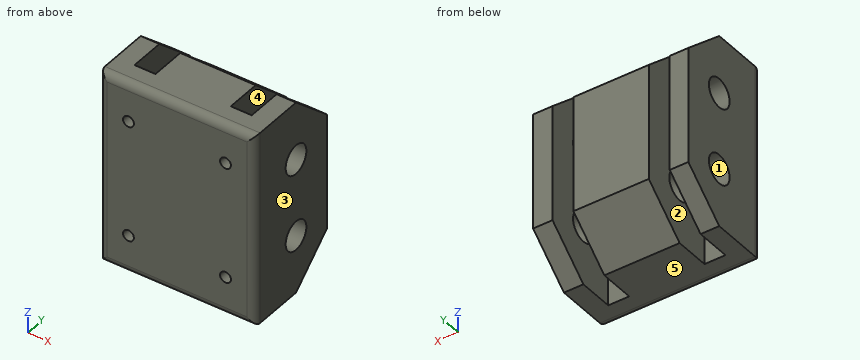
```python
from build123d import *

# Parameters (mm, degrees)
SKETCH1_W           = 63.5
SKETCH1_H           = 6.35
BOSS_EXTRUDE1_DEPTH = 50.8
BOSS_EXTRUDE2_DEPTH = 50.8
SKETCH10_W          = 6.858
SKETCH10_H          = 25.629031657
CUT_EXTRUDE1_DEPTH  = 88.854357354
LPATTERN3_COUNT     = 2
LPATTERN3_PITCH     = 31.496
SKETCH11_R          = 4.7625
CUT_EXTRUDE2_DEPTH  = 88.854357354
FILLET1_R           = 2.54
SKETCH19_R          = 1.778
CUT_EXTRUDE3_DEPTH  = 7.62


with BuildPart() as part:
    # Sketch1 → Boss-Extrude1 (new body)
    with BuildSketch(Plane(origin=(0, 0, 0), x_dir=(0, 0, -1), z_dir=(1, 0, 0))):
        with Locations((31.75, 3.175)):
            Rectangle(SKETCH1_W, SKETCH1_H)
    extrude(amount=-BOSS_EXTRUDE1_DEPTH)

    # Sketch2 → Boss-Extrude2 (add)
    with BuildSketch(Plane(origin=(0, 0, 0), x_dir=(0, 0, -1), z_dir=(1, 0, 0))):
        Polygon((0, 6.35), (0, 19.05), (12.7, 33.249031657), (50.8, 33.249031657), (63.5, 19.05), (63.5, 6.35), align=None)
    extrude(amount=-BOSS_EXTRUDE2_DEPTH)

    # Sketch10 → Cut-Extrude1 (cut, through all)
    with BuildSketch(Plane(origin=(0, 0, -63.5), x_dir=(-1, 0, 0), z_dir=(0, 0, -1))):
        with Locations((9.779, 20.434515829)):
            Rectangle(SKETCH10_W, SKETCH10_H)
    cut_extrude1 = extrude(amount=-CUT_EXTRUDE1_DEPTH, mode=Mode.SUBTRACT)

    # LPattern3: Cut-Extrude1 ×2
    with Locations(*[(-i * LPATTERN3_PITCH, 0, 0) for i in range(1, LPATTERN3_COUNT)]):
        add(cut_extrude1, mode=Mode.SUBTRACT)

    # Sketch11 → Cut-Extrude2 (cut, through all)
    with BuildSketch(Plane(origin=(0, 0, 0), x_dir=(0, 0, -1), z_dir=(1, 0, 0))):
        with Locations((19.05, 19.05)):
            Circle(SKETCH11_R)
        with Locations((44.45, 19.05)):
            Circle(SKETCH11_R)
    extrude(amount=-CUT_EXTRUDE2_DEPTH, mode=Mode.SUBTRACT)

    # Fillet1
    fillet1_edges = [part.edges().sort_by_distance(p)[0] for p in [
        (0, 0, -31.75),
        (-50.8, 0, -31.75),
        (-25.4, 0, -63.5),
        (-25.4, 0, 0),
    ]]
    fillet(fillet1_edges, radius=FILLET1_R)

    # Sketch19 → Cut-Extrude3 (cut)
    with BuildSketch(Plane.XZ):
        with Locations(Location((-9.525, -50.8, 0), (0, 0, 270))):
            Circle(SKETCH19_R)
        with Locations(Location((-41.275, -50.8, 0), (0, 0, 270))):
            Circle(SKETCH19_R)
        with Locations(Location((-41.275, -12.7, 0), (0, 0, 270))):
            Circle(SKETCH19_R)
        with Locations(Location((-9.525, -12.7, 0), (0, 0, 270))):
            Circle(SKETCH19_R)
    extrude(amount=-CUT_EXTRUDE3_DEPTH, mode=Mode.SUBTRACT)


solid = part.part
```
For this review, take the finished solid that the model builds, in its own axes (mm). Face numbers are marked on the shaded views. A direction names the side the tool comes from. Coordinates: 2 decimals unless noted, no trailing zeros. Write each loop counter-clockwise with the first axis right and the second up, starting at its lowest first coordinate (ties: lowest second). Pieces come first, ordered by that corner, then holes. Notation, with made-up numbers: (16, -13.5) - (68, -13.5) arc R23 cw to (68, 3.5) - close; hole circle Ø9 at (-2, 6). An arc over 180 degrees is marked (long way). Answer in a Markdown table with one row per item. Add a question column.
Q1. For probe 1 along X at (y, z) = (22, -57); probe 2 along X at (y, z) = (4.5, -50.8); probe 3 along Y at (x, z) = (-19.25, -19.05), list the stretches that pass through material, from the lowest coordinate up.
Q2. Tool access review of the marked faces 1 and 2: name each direction out of +Z, -Z, +X, -X, +Y, -Y from which nothing blocks a thin tool from reaching the whole face with its end or side.
Q3. We need section B-B, the plane x = -23.5. Count the separate pieces of the cut face and the enclosed holes in it, and give its area (3 significant figures).
Q4. For P1, Ø8, axis at y = 18, z = -55, coming from the +X side; P2, Ø2, axis at x = -29.5, y = 27, coming from the -Z side; P3, Ø3.5, axis at x = -41.5, z = -17, coming from the +Y side, all flat-tipped, find the tip position at first contact; note any pin that passes through.
Q5. We need section C-C, the plane y = 27. State the section outline as (x, z) points.
Q6. We need section A-A, the plane z = -44.45. State the section outline as (x, y) points.
Q7. Draft analysis for pull direction X (two halves, no side actions). For the marked faces 3, 4 and 5, state which applies: +X half, -X half, draft (parallel to the pull), parting line (faces both ways), or undercut.
Q8. We need section D-D, the plane z = -32.5. State the section outline as (x, y) points, and give its area (3 significant figures).
Answer list:
| question | item | result |
|---|---|---|
| 1 | probe 1 | x = -50.8 to -44.7, -37.85 to -13.21, -6.35 to 0 |
| 1 | probe 2 | x = -50.8 to -43.05, -39.5 to -11.3, -7.75 to 0 |
| 1 | probe 3 | y = 0 to 14.29, 23.81 to 33.25 |
| 2 | face 1 | +X, -X |
| 2 | face 2 | +Z, -Z, +Y |
| 3 | separate pieces | 1 |
| 3 | enclosed holes | 2 |
| 3 | area | 1,790 mm2 |
| 4 | P1 | stops at x = 0 |
| 4 | P2 | stops at z = -57.28 |
| 4 | P3 | stops at y = 7.62 |
| 5 | outline | (-50.8, -56.39) - (-44.7, -56.39) - (-44.7, -7.11) - (-50.8, -7.11) - close; (-37.85, -56.39) - (-13.21, -56.39) - (-13.21, -7.11) - (-37.85, -7.11) - close; (-6.35, -56.39) - (0, -56.39) - (0, -7.11) - (-6.35, -7.11) - close |
| 6 | outline | (-50.8, 2.54) arc R2.54 ccw to (-48.26, 0) - (-2.54, 0) arc R2.54 ccw to (0, 2.54) - (0, 14.29) - (-6.35, 14.29) - (-6.35, 7.62) - (-13.21, 7.62) - (-13.21, 14.29) - (-37.85, 14.29) - (-37.85, 7.62) - (-44.7, 7.62) - (-44.7, 14.29) - (-50.8, 14.29) - close; (-50.8, 23.81) - (-44.7, 23.81) - (-44.7, 33.25) - (-50.8, 33.25) - close; (-37.85, 23.81) - (-13.21, 23.81) - (-13.21, 33.25) - (-37.85, 33.25) - close; (-6.35, 23.81) - (0, 23.81) - (0, 33.25) - (-6.35, 33.25) - close |
| 7 | face 3 | +X half |
| 7 | face 4 | undercut |
| 7 | face 5 | draft |
| 8 | outline | (-50.8, 2.54) arc R2.54 ccw to (-48.26, 0) - (-2.54, 0) arc R2.54 ccw to (0, 2.54) - (0, 33.25) - (-6.35, 33.25) - (-6.35, 7.62) - (-13.21, 7.62) - (-13.21, 33.25) - (-37.85, 33.25) - (-37.85, 7.62) - (-44.7, 7.62) - (-44.7, 33.25) - (-50.8, 33.25) - close |
| 8 | area | 1,330 mm2 |
